Model file for the job. Use its own axes, mm. Face numbers are marked on the shaded views. A direction names the side the tool comes from. Coordinates: 2 decimals unless noted, no trailing zeros. Loops run counter-clockwise (first coordinate to the right, second up) from the corner with the lowest first, then second, coordinate; pieces in that order, holes last. Notation, with made-up numbers: (16.5, -7) - (68.5, -7) arc R32 ccw to (68.5, 32) - close; hole circle Ø2 at (76, 36.25). An arc over 180 degrees is marked (long way). Write each question's results on one line, items separated by ' | '. Start each with the question number.
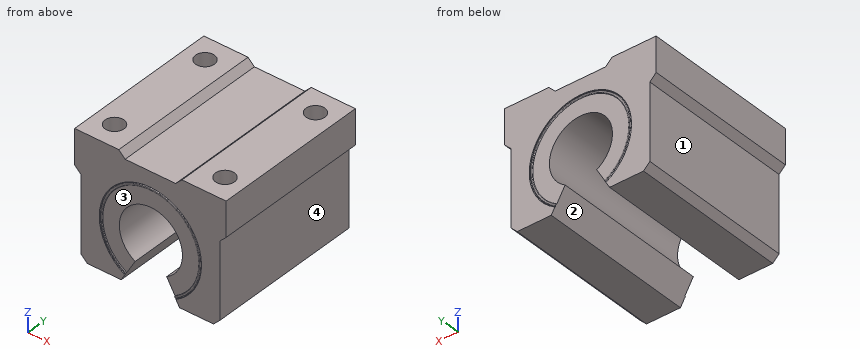
```python
from build123d import *

# Parameters (mm, degrees)
EXTRUDE_2_DEPTH     = 50
CHAMFER_1_SIZE      = 2
SKETCH_5_R          = 3
CUT_EXTRUDE_1_DEPTH = 12
CHAMFER_2_SIZE      = 2


with BuildPart() as part:
    # 草图4 → 拉伸2 (new body)
    with BuildSketch(Plane(origin=(0, -25, 0), x_dir=(-1, 0, 0), z_dir=(0, 1, 0))):
        with BuildLine():
            Line((8, 21), (-8, 21))
            Line((-8, 21), (-8, 23))
            Line((-8, 23), (-24, 23))
            Line((-24, 23), (-24, 12))
            Line((-24, 12), (-22, 10))
            Line((-22, 10), (-22, -16))
            Line((-22, -16), (-9.237604307, -16))
            Line((-9.237604307, -16), (-5, -8.660254038))
            ThreePointArc((-5, -8.660254038), (0, 10), (5, -8.660254038))
            Line((5, -8.660254038), (9.237604307, -16))
            Line((9.237604307, -16), (22, -16))
            Line((22, -16), (22, 10))
            Line((22, 10), (24, 12))
            Line((24, 12), (24, 23))
            Line((24, 23), (8, 23))
            Line((8, 23), (8, 21))
        make_face()
    extrude(amount=EXTRUDE_2_DEPTH)

    # 倒角1
    chamfer_1_edges = [part.edges().sort_by_distance(p)[0] for p in [
        (-8, 0, 23),
        (8, 0, 23),
    ]]
    chamfer(chamfer_1_edges, length=CHAMFER_1_SIZE - 0.0001)  # a hair under: the kernel refuses the full size

    # 草图5 → 切除-拉伸1 (cut)
    with BuildSketch(Plane.XY.offset(23)):
        with Locations((-17.5, 17.5)):
            Circle(SKETCH_5_R)
        with Locations((17.5, 17.5)):
            Circle(SKETCH_5_R)
        with Locations((17.5, -17.5)):
            Circle(SKETCH_5_R)
        with Locations((-17.5, -17.5)):
            Circle(SKETCH_5_R)
    extrude(amount=-CUT_EXTRUDE_1_DEPTH, mode=Mode.SUBTRACT)

    # 倒角2
    chamfer_2_edges = [part.edges().sort_by_distance(p)[0] for p in [
        (-22, 0, -16),
        (22, 0, -16),
    ]]
    chamfer(chamfer_2_edges, length=CHAMFER_2_SIZE)

    # 草图6 → 切除-旋转1 (revolve, cut)
    with BuildSketch(Plane(origin=(0, 0, 0), x_dir=(0, 0, -1), z_dir=(1, 0, 0))):
        with BuildLine():
            Line((-16.2, -25), (-16, -24.8))
            ThreePointArc((-16, -24.8), (-15.940621125, -24.941496067), (-15.798761062, -25))
            Line((-15.798761062, -25), (-16.2, -25))
        make_face()
        with BuildLine():
            Line((-15.45, -25), (0, -25))
            Line((0, -25), (0, -24.8))
            Line((0, -24.8), (-15.25, -24.8))
            ThreePointArc((-15.25, -24.8), (-15.308578644, -24.941421356), (-15.45, -25))
        make_face()
    cut_revolve_1 = revolve(axis=Axis((0, -10.264906919, 0), (0, -1, 0)), mode=Mode.SUBTRACT)

    # 镜向1: 切除-旋转1 across plane
    add(cut_revolve_1.mirror(Plane.ZX), mode=Mode.SUBTRACT)


solid = part.part
```
Q1. Pin check, flat tips, straight feed: pin 1 (6 mm diameter, centred on y = 9.5, z = 8, fed in from -X); pin 2 (12 mm diameter, centred on x = -3, z = -7, fed in from +Y); pin 3 (1.8 mm diameter, centred on x = -18, y = -18.5, fed in from +Z); pin 4 (5 mm diameter, centred on x = 17, y = -16, fed in from +Z). Stop position of each tip, or through.
Q2. Which spindle directions (+Z, -Z, +X, -X, +Y, -Y) get a long thin tool onto all of the face, cutting with end or side? Do the marked faces 1, 2, 3 and 4. Say none if no direction does.
Q3. Cut at D-D (x = -17.5). List the corners of the cut face in (y, z).
Q4. Drill centre lines: L1, parallel to Y at x = 17.5, z = 14; L2, parallel to X at y = -17, z = 19; L3, parallel to Y at x = -5, z = 13.5. Where is each one in solid material? Low to high. Write a range as from..to.
Q5. Cut at B-B (x = 0). List the corners of the cut face in (y, z), and give its area (3 significant figures).
Q6. Cut at A-A (z = 17). List the corners of the cut face in (x, y).
Check result:
1) pin 1: x = -23 | pin 2: y = 24.8 | pin 3: z = 11 | pin 4: z = 23
2) face 1: -Z, -X, +Y, -Y | face 2: -Z, +Y, -Y | face 3: -Y | face 4: -Z, +X, +Y, -Y
3) outline: (-25, -16) - (25, -16) - (25, 23) - (20.5, 23) - (20.5, 11) - (14.5, 11) - (14.5, 23) - (-14.5, 23) - (-14.5, 11) - (-20.5, 11) - (-20.5, 23) - (-25, 23) - close
4) L1: -25..-20.5, -14.5..14.5, 20.5..25 | L2: -24..-20.46, -14.54..14.54, 20.46..24 | L3: -24.8..24.8
5) outline: (-25, 15.45) arc R0.2 ccw to (-24.8, 15.25) - (-24.8, 10) - (24.8, 10) - (24.8, 15.25) arc R0.2 ccw to (25, 15.45) - (25, 15.8) arc R0.2 ccw to (24.8, 16) - (25, 16.2) - (25, 21) - (-25, 21) - (-25, 16.2) - (-24.8, 16) arc R0.2 ccw to (-25, 15.8) - close | area: 548 mm²
6) outline: (-24, -25) - (24, -25) - (24, 25) - (-24, 25) - close; hole circle Ø6 at (-17.5, -17.5); hole circle Ø6 at (-17.5, 17.5); hole circle Ø6 at (17.5, -17.5); hole circle Ø6 at (17.5, 17.5)
